```python
from build123d import *

# Parameters (mm, degrees)
SKETCH1_W           = 76.2
SKETCH1_H           = 25.4
BOSS_EXTRUDE1_DEPTH = 9.525
SKETCH2_R           = 2.159
CUT_EXTRUDE1_DEPTH  = 42.275
SKETCH3_R           = 3.302
CUT_EXTRUDE2_DEPTH  = 1.27
SKETCH4_R           = 0.79375
CUT_EXTRUDE3_DEPTH  = 42.275
SKETCH5_R           = 3.302
CUT_EXTRUDE4_DEPTH  = 78.836081768


with BuildPart() as part:
    # Sketch1 → Boss-Extrude1 (new body)
    with BuildSketch(Plane(origin=(0, 0, 0), x_dir=(1, 0, 0), z_dir=(0, 1, 0))):
        Rectangle(SKETCH1_W, SKETCH1_H)
    extrude(amount=BOSS_EXTRUDE1_DEPTH)

    # Sketch2 → Cut-Extrude1 (cut, through all)
    with BuildSketch(Plane(origin=(0, 9.525, 0), x_dir=(1, 0, 0), z_dir=(0, 1, 0))):
        with Locations(Location((-32.074075882, 7.9375, 0), (0, 0, 270))):
            Circle(SKETCH2_R)
        with Locations(Location((-32.074075882, -7.9375, 0), (0, 0, 270))):
            Circle(SKETCH2_R)
        with Locations(Location((31.425924118, 7.9375, 0), (0, 0, 270))):
            Circle(SKETCH2_R)
        with Locations(Location((31.425924118, -7.9375, 0), (0, 0, 270))):
            Circle(SKETCH2_R)
    extrude(amount=-CUT_EXTRUDE1_DEPTH, mode=Mode.SUBTRACT)

    # Sketch3 → Cut-Extrude2 (cut)
    with BuildSketch(Plane(origin=(0, 9.525, 0), x_dir=(1, 0, 0), z_dir=(0, 1, 0))):
        with Locations(Location((-9.525, 7.9375, 0), (0, 0, 270))):
            Circle(SKETCH3_R)
        with Locations(Location((-9.525, -7.9375, 0), (0, 0, 270))):
            Circle(SKETCH3_R)
        with Locations(Location((9.525, -7.9375, 0), (0, 0, 270))):
            Circle(SKETCH3_R)
        with Locations(Location((9.525, 7.9375, 0), (0, 0, 270))):
            Circle(SKETCH3_R)
    extrude(amount=-CUT_EXTRUDE2_DEPTH, mode=Mode.SUBTRACT)

    # Sketch4 → Cut-Extrude3 (cut, through all)
    with BuildSketch(Plane(origin=(0, 9.525, 0), x_dir=(1, 0, 0), z_dir=(0, 1, 0))):
        with Locations(Location((-15.875, 7.9375, 0), (0, 0, 270))):
            Circle(SKETCH4_R)
        with Locations(Location((-15.875, -7.9375, 0), (0, 0, 270))):
            Circle(SKETCH4_R)
        with Locations(Location((3.175, 6.35, 0), (0, 0, 270))):
            Circle(SKETCH4_R)
        with Locations(Location((3.175, -6.35, 0), (0, 0, 270))):
            Circle(SKETCH4_R)
    extrude(amount=-CUT_EXTRUDE3_DEPTH, mode=Mode.SUBTRACT)

    # Sketch5 → Cut-Extrude4 (cut, through all)
    with BuildSketch(Plane.ZY.offset(38.1)):
        with Locations((0, 9.525)):
            Circle(SKETCH5_R)
    extrude(amount=-CUT_EXTRUDE4_DEPTH, mode=Mode.SUBTRACT)


solid = part.part
```
Input: part model. Units: mm. Frame: model coordinates. A direction names the side the tool comes from. Give positions to 0.01 mm unless a question says otherwise; leave off trailing zeros. Order: outer loops, then holes, each group sorted by start corner. A loop starts at its lowest first (then second) coordinate and runs counter-clockwise, first axis right, second up. Notation, with made-up numbers: (-15.5, 10.25) - (8.5, 10.25) arc R32 cw to (8.5, 39.25) - close; hole circle Ø10 at (-23, -17). An arc over 180 degrees is marked (long way). Put each result on its own line as item: value.
Item 1: Ray query, L1, parallel to X at y = 4.5, z = 9.5; L2, parallel to Z at x = -8, y = 9; L3, parallel to X at y = 4.25, z = -6.35. Return the intervals inside material, ascending. Write a range as from..to.
Found:
L1: x = -38.1..-33.56, -30.58..29.94, 32.92..38.1
L2: z = -12.7..-10.87, -5.01..-3.26, 3.26..5.01, 10.87..12.7
L3: x = -38.1..-33.54, -30.61..2.38, 3.97..29.96, 32.89..38.1
Item 2: Draft query along Z for faces 1 (the flat face through (-1, 0, 0)), 2 (the flat face through (10, 8.255, 8)). Return one class per face: +Z half, -Z half, draft (parallel to the pull), parting line (faces both ways), or undercut.
Found:
face 1: draft
face 2: undercut
Item 3: Section query D-D, the plane z = 0. Return loops of the section in (x, y).
Found:
outline: (-38.1, 0) - (38.1, 0) - (38.1, 6.22) - (-38.1, 6.22) - close
Item 4: Contact query for flat-ended pins moving along their axis: pin 1 (1 mm diameter, centred on x = -0.5, z = 4, fed in from -Y); pin 2 (2.5 mm diameter, centred on x = -32.07, z = 7.94, fed in from -Y); pin 3 (3.5 mm diameter, centred on x = 8.5, z = -7.5, fed in from +Y) (3 decimals); pin 4 (4 mm diameter, centred on x = 21, z = 0.5, fed in from +Y). Output: stop coordinate, or through.
Found:
pin 1: stops at y = 0
pin 2: passes through
pin 3: stops at y = 8.255
pin 4: stops at y = 7.37
Item 5: Section query C-C, the plane x = -8. Return loops of the section in (y, z) (3 decimals).
Found:
outline: (0, -12.7) - (9.525, -12.7) - (9.525, -10.866) - (8.255, -10.866) - (8.255, -5.009) - (9.525, -5.009) - (9.525, -3.302) arc R3.302 cw to (9.525, 3.302) - (9.525, 5.009) - (8.255, 5.009) - (8.255, 10.866) - (9.525, 10.866) - (9.525, 12.7) - (0, 12.7) - close
Item 6: Access query for faces 3 (the flat face through (-1, 9.525, 8)), 4 (the cylindrical face through (6.3, 8.9, 7.22)). Directions: +Z, -Z, +X, -X, +Y, -Y. A direction counts if a zero-diameter tool reaches every point of the face in a straight line with its end or side. Return the directions, or none.
Found:
face 3: +Z, -Z, +X, -X, +Y
face 4: +Y
Item 7: Section query A-A, the plane y = 7.5. Count the separate pieces of the cut face and the enclosed holes in it, then the cut area to 3 significant figures.
Found:
separate pieces: 2
enclosed holes: 8
area: 1,470 mm^2
